The listing builds one solid part. Answer for the finished solid, in the listing's coordinates (mm). Face numbers are marked on the shaded views. A direction names the side the tool comes from. Give positions to 0.01 mm unless a question says otherwise; leave off trailing zeros. Write each loop counter-clockwise with the first axis right and the second up, starting at its lowest first coordinate (ties: lowest second). Pieces come first, ordered by that corner, then holes. Notation, with made-up numbers: (24.5, -10.75) - (63.5, -10.75) arc R31 cw to (63.5, 21.25) - close; hole circle Ø10 at (43.25, 41). An arc over 180 degrees is marked (long way). Answer as CSV lines item,"result". Start each with the question number.
(1) Find section A-A (z = 3.5). Write down the section's boundary in (x, y), then the cut area to 3 significant figures.
(2) For the marked faces 4, 5, 6 and 7, determine the directions among +Z, -Z, +X, -X, +Y, -Y from which every point of the face is accessible in a straight line to the end or side of a thin tool.
(3) Find section B-B (y = -11). Write down the section's boundary in (x, z).
(4) Straight lines are drawn through the part: probe 1 along X at (y, z) = (-5.15, 9); probe 2 along X at (y, z) = (-28, 8.75); probe 3 along X at (y, z) = (-31.8, 9). For each, find the intervals that lie inside material, in ascending order.
(5) Find section D-D (z = 8). State how many separate pieces and enclosed holes the cut face has, then the cut area to 3 significant figures.
(6) Find section C-C (x = -32.5). Write down the section's boundary in (y, z).
(7) For a pull along X with two mould halves and no side action, classify the marked faces 1, 2 and 3 as pulls with the +X half, pulls with the -X half, needs draft (parallel to the pull), parting line crosses it, or undercut.
(8) Each of these flat-tipped pins is pushed along its axis until it touches: pin 1 Ø4 at (y, z) = (-31, 12) entering from +X; pin 2 Ø2.5 at (x, y) = (-4.5, -6) entering from +Z; pin 3 Ø5 at (y, z) = (-19.5, 5.5) entering from -X; pin 4 Ø3.5 at (x, y) = (-16, -3) entering from +Z. Where does it stop, or does it pass through?
from build123d import *

# Parameters (mm, degrees)
CROQUIS1_W              = 25
CROQUIS1_H              = 34
SALIENTE_EXTRUIR1_DEPTH = 6
CROQUIS2_W              = 7
CROQUIS2_H              = 5
SALIENTE_EXTRUIR2_DEPTH = 6
CORTAR_EXTRUIR1_REACH   = 44.626
CROQUIS3_W              = 11
CROQUIS3_H              = 26
REDONDEO1_R             = 4
SALIENTE_EXTRUIR3_DEPTH = 12
SALIENTE_EXTRUIR4_DEPTH = 2
CORTAR_EXTRUIR2_REACH   = 70.45
CROQUIS7_R              = 1.75
CORTAR_EXTRUIR3_REACH   = 67.577
CROQUIS8_W              = 27.3
CROQUIS8_H              = 5


with BuildPart() as part:
    # Croquis1 → Saliente-Extruir1 (new body)
    with BuildSketch(Plane.XY):
        with Locations((-12.5, -17)):
            Rectangle(CROQUIS1_W, CROQUIS1_H)
    extrude(amount=SALIENTE_EXTRUIR1_DEPTH)

    # Croquis2 → Saliente-Extruir2 (add)
    with BuildSketch(Plane.XY.offset(6)):
        with Locations((-21.5, -5.5)):
            Rectangle(CROQUIS2_W, CROQUIS2_H)
        with Locations((-3.5, -5.5)):
            Rectangle(CROQUIS2_W, CROQUIS2_H)
        with Locations((-3.5, -31.5)):
            Rectangle(CROQUIS2_W, CROQUIS2_H)
        with Locations((-21.5, -31.5)):
            Rectangle(CROQUIS2_W, CROQUIS2_H)
    extrude(amount=SALIENTE_EXTRUIR2_DEPTH)

    # Croquis3 → Cortar-Extruir1 (cut, up to next)
    with BuildSketch(Plane.XY.offset(6), mode=Mode.PRIVATE) as cortar_extruir1_sk1:
        with Locations((-12.5, -16)):
            Rectangle(CROQUIS3_W, CROQUIS3_H)
    cortar_extruir1_tool1 = extrude(cortar_extruir1_sk1.sketch, amount=-CORTAR_EXTRUIR1_REACH, mode=Mode.PRIVATE) & part.part
    add(cortar_extruir1_tool1.solids().sort_by_distance((-12.5, -16, 6))[0], mode=Mode.SUBTRACT)

    # Redondeo1
    # the kernel refuses this fillet: 4 mm, written as the material it adds along each edge
    with BuildSketch(Plane(origin=(-18, -29, 6), x_dir=(0, 1, 0), z_dir=(0, 0, -1)), Plane(origin=(-7, -29, 6), x_dir=(-1, 0, 0), z_dir=(0, 0, -1)), Plane(origin=(-18, -3, 6), x_dir=(1, 0, 0), z_dir=(0, 0, -1))) as redondeo1_piece_1:
        with BuildLine():
            CenterArc((REDONDEO1_R, REDONDEO1_R), REDONDEO1_R, 180, 90)
            Line((0, REDONDEO1_R), (0, 0))
            Line((0, 0), (REDONDEO1_R, 0))
        make_face()
    extrude(amount=6)
    with BuildSketch(Plane(origin=(-7, -3, 6), x_dir=(-1, 0, 0), z_dir=(0, 0, -1))) as redondeo1_piece_2:
        with BuildLine():
            CenterArc((REDONDEO1_R, -REDONDEO1_R), REDONDEO1_R, 90, 90)
            Line((0, -REDONDEO1_R), (0, 0))
            Line((0, 0), (REDONDEO1_R, 0))
        make_face()
    extrude(amount=6)
    # the kernel refuses this fillet: 4 mm, written as the material it takes off along each edge
    with BuildSketch(Plane(origin=(0, 0, -10), x_dir=(-1, 0, 0), z_dir=(0, 0, 1))) as redondeo1_2_piece_1:
        with BuildLine():
            CenterArc((REDONDEO1_R, REDONDEO1_R), REDONDEO1_R, 180, 90)
            Line((0, REDONDEO1_R), (0, 0))
            Line((0, 0), (REDONDEO1_R, 0))
        make_face()
    extrude(amount=26, mode=Mode.SUBTRACT)
    with BuildSketch(Plane(origin=(0, -34, 22), x_dir=(0, 1, 0), z_dir=(0, 0, -1)), Plane(origin=(-25, -34, -10), x_dir=(0, 1, 0), z_dir=(0, 0, 1))) as redondeo1_2_piece_2:
        with BuildLine():
            CenterArc((REDONDEO1_R, -REDONDEO1_R), REDONDEO1_R, 90, 90)
            Line((0, -REDONDEO1_R), (0, 0))
            Line((0, 0), (REDONDEO1_R, 0))
        make_face()
    extrude(amount=32, mode=Mode.SUBTRACT)
    with BuildSketch(Plane(origin=(-25, 0, -10), x_dir=(1, 0, 0), z_dir=(0, 0, 1))) as redondeo1_2_piece_3:
        with BuildLine():
            CenterArc((REDONDEO1_R, -REDONDEO1_R), REDONDEO1_R, 90, 90)
            Line((0, -REDONDEO1_R), (0, 0))
            Line((0, 0), (REDONDEO1_R, 0))
        make_face()
    extrude(amount=26, mode=Mode.SUBTRACT)

    # Croquis5 → Saliente-Extruir3 (add)
    with BuildSketch(Plane(origin=(0, 0, 0), x_dir=(-1, 0, 0), z_dir=(0, 0, -1))):
        with BuildLine():
            Line((25, -29), (25, -30))
            ThreePointArc((25, -30), (23.828427125, -32.828427125), (21, -34))
            Line((21, -34), (25, -34))
            Line((25, -34), (59.4, -34))
            Line((59.4, -34), (59.4, -24))
            Line((59.4, -24), (25, -24))
            Line((25, -24), (25, -29))
        make_face()
    extrude(amount=-SALIENTE_EXTRUIR3_DEPTH)

    # Croquis6 → Saliente-Extruir4 (add)
    with BuildSketch(Plane.XY.offset(12)):
        Polygon((-18, -29), (-25, -29), (-25, -24), (-59.4, -24), (-59.4, -34), (-18, -34), align=None)
    extrude(amount=SALIENTE_EXTRUIR4_DEPTH)

    # Cortar-Extruir2: up to this face of the body (flat: up to its plane)
    cortar_extruir2_end = Plane(part.part.faces().sort_by_distance((-34.409507042, -34, 6.559859155))[0])
    # Croquis7 → Cortar-Extruir2 (cut, up to the picked face)
    with BuildSketch(Plane(origin=(0, -3, 0), x_dir=(1, 0, 0), z_dir=(0, 1, 0)), mode=Mode.PRIVATE) as cortar_extruir2_sk1:
        with Locations(Location((-21.772983346, -9, 0), (0, 0, 270))):
            Circle(CROQUIS7_R)
    cortar_extruir2_tool1 = split(extrude(cortar_extruir2_sk1.sketch, amount=-CORTAR_EXTRUIR2_REACH, mode=Mode.PRIVATE), bisect_by=cortar_extruir2_end, keep=Keep.BOTH, mode=Mode.PRIVATE)
    # Croquis7 → Cortar-Extruir2 (cut, up to the picked face)
    with BuildSketch(Plane(origin=(0, -3, 0), x_dir=(1, 0, 0), z_dir=(0, 1, 0)), mode=Mode.PRIVATE) as cortar_extruir2_sk2:
        with Locations(Location((-3.227016654, -9, 0), (0, 0, 243.787297197))):
            Circle(CROQUIS7_R)
    cortar_extruir2_tool2 = split(extrude(cortar_extruir2_sk2.sketch, amount=-CORTAR_EXTRUIR2_REACH, mode=Mode.PRIVATE), bisect_by=cortar_extruir2_end, keep=Keep.BOTH, mode=Mode.PRIVATE)
    add(cortar_extruir2_tool1.solids().sort_by(Axis((-21.772983, -3, 9), (0, -1, 0)))[0], mode=Mode.SUBTRACT)
    add(cortar_extruir2_tool2.solids().sort_by(Axis((-3.227017, -3, 9), (0, -1, 0)))[0], mode=Mode.SUBTRACT)

    # Croquis8 → Cortar-Extruir3 (cut, up to next)
    with BuildSketch(Plane(origin=(0, -24, 0), x_dir=(1, 0, 0), z_dir=(0, 1, 0)), mode=Mode.PRIVATE) as cortar_extruir3_sk1:
        with Locations((-42.2, -7)):
            Rectangle(CROQUIS8_W, CROQUIS8_H)
    cortar_extruir3_tool1 = extrude(cortar_extruir3_sk1.sketch, amount=-CORTAR_EXTRUIR3_REACH, mode=Mode.PRIVATE) & part.part
    add(cortar_extruir3_tool1.solids().sort_by_distance((-42.2, -24, 7))[0], mode=Mode.SUBTRACT)


solid = part.part
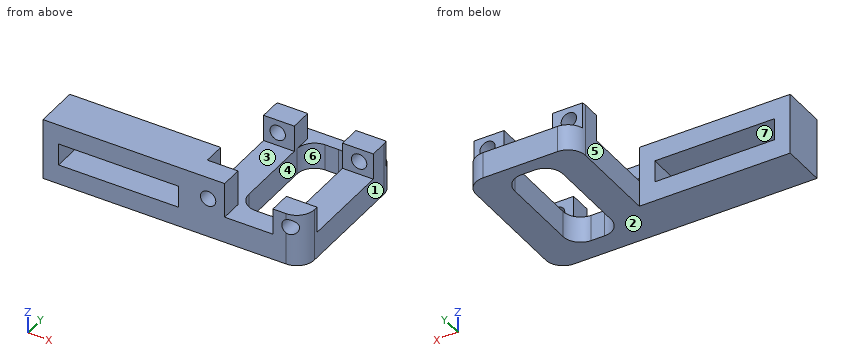
Result set:
1,outline,"(-59.4, -34) - (-4, -34) arc R4 ccw to (0, -30) - (0, -4) arc R4 ccw to (-4, 0) - (-21, 0) arc R4 ccw to (-25, -4) - (-25, -24) - (-59.4, -24) - close; hole (-18, -25) arc R4 ccw to (-14, -29) - (-11, -29) arc R4 ccw to (-7, -25) - (-7, -7) arc R4 ccw to (-11, -3) - (-14, -3) arc R4 ccw to (-18, -7) - close"
1,area,"911 mm^2"
2,face 4,"+Z"
2,face 5,"+Z, -Z, -X, +Y"
2,face 6,"+Z, -Z"
2,face 7,"+Y, -Y"
3,outline,"(-25, 0) - (-18, 0) - (-18, 6) - (-25, 6) - close; (-7, 0) - (0, 0) - (0, 6) - (-7, 6) - close"
4,probe 1,"-25 to -23.52, -20.02 to -18, -7 to -4.98, -1.48 to 0"
4,probe 2,"-59.4 to -55.85, -28.55 to -25"
4,probe 3,"-59.4 to -55.85, -28.55 to -23.52, -20.02 to -18, -7 to -4.98, -1.48 to -0.43"
5,separate pieces,"9"
5,enclosed holes,"0"
5,area,"151 mm^2"
6,outline,"(-34, 0) - (-24, 0) - (-24, 4.5) - (-34, 4.5) - close; (-34, 9.5) - (-24, 9.5) - (-24, 14) - (-34, 14) - close"
7,face 1,"pulls with the +X half"
7,face 2,"needs draft"
7,face 3,"undercut"
8,pin 1,"x = 0"
8,pin 2,"z = 12"
8,pin 3,"x = -25"
8,pin 4,"z = 6"
